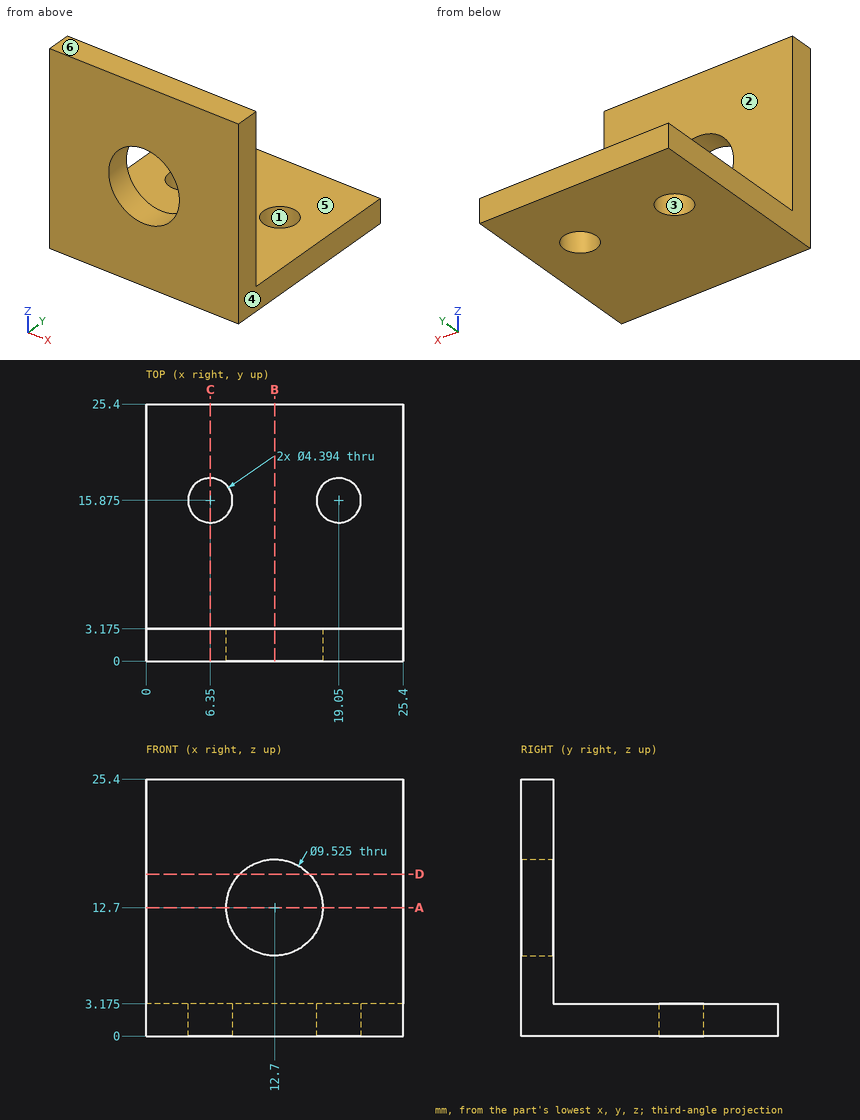
Job drawing, mm, ordinate dimensions from the low corner. One solid piece. A direction names the side the tool comes from. Round coordinates to 2 decimals unless told otherwise and drop trailing zeros. Loops run counter-clockwise (first coordinate to the right, second up) from the corner with the lowest first, then second, coordinate; pieces in that order, holes last.
(1) Two-plate mould, pull along Y, no slides. Class the marked faces 1, 2, 3 and 4: +Y half, -Y half, draft (parallel to the pull), parting line (faces both ways), or undercut.
(2) Cut at C-C (x = 6.35). Give the cut face in (y, z) (1 decimal), plus the area to 3 significant figures.
(3) Drop flat-ended pins along their axis: pin 1 (4 mm diameter, centred on y = 3, z = 6, fed in from -X); pin 2 (3 mm diameter, centred on x = 9.5, z = 11, fed in from +Y) (3 decimals); pin 3 (10 mm diameter, centred on x = 17, y = 16.5, fed in from +Z) (3 decimals). Give the stop position or say it passes through.
(4) Cut at B-B (x = 12.7). Give the cut face in (y, z) (1 decimal), plus the area to 3 significant figures.
(5) Which spindle directions (+Z, -Z, +X, -X, +Y, -Y) get a long thin tool onto all of the face, cutting with end or side? Do the marked faces 5 and 6. Say none if no direction does.
(6) Wall check: line 1 along Y through (x, z) = (6.35, 0.75); line 2 along Z through (x, y) = (12.7, 1.8); line 3 along X through (y, z) = (17.5, 2.25). Give the ranges that are in metal, low to high.
(7) Cut at D-D (z = 16). Give the cut face in (x, y) (1 decimal).
(8) Cut at A-A (z = 12.7). Give the cut face in (x, y) (1 decimal).
Findings below:
1. face 1: undercut
1. face 2: +Y half
1. face 3: undercut
1. face 4: draft
2. outline: (0, 0) - (13.7, 0) - (13.7, 3.2) - (3.2, 3.2) - (3.2, 25.4) - (0, 25.4) - close; (18.1, 0) - (25.4, 0) - (25.4, 3.2) - (18.1, 3.2) - close
2. area: 137 mm2
3. pin 1: stops at x = 0
3. pin 2: stops at y = 3.175
3. pin 3: stops at z = 3.175
4. outline: (0, 0) - (25.4, 0) - (25.4, 3.2) - (3.2, 3.2) - (3.2, 7.9) - (0, 7.9) - close; (0, 17.5) - (3.2, 17.5) - (3.2, 25.4) - (0, 25.4) - close
4. area: 121 mm2
5. face 5: +Z, +X, -X, +Y
5. face 6: +Z, +X, -X, +Y, -Y
6. line 1: y = 0 to 13.68, 18.07 to 25.4
6. line 2: z = 0 to 7.94, 17.46 to 25.4
6. line 3: x = 0 to 4.87, 7.83 to 17.57, 20.53 to 25.4
7. outline: (0, 0) - (9.3, 0) - (9.3, 3.2) - (0, 3.2) - close; (16.1, 0) - (25.4, 0) - (25.4, 3.2) - (16.1, 3.2) - close
8. outline: (0, 0) - (7.9, 0) - (7.9, 3.2) - (0, 3.2) - close; (17.5, 0) - (25.4, 0) - (25.4, 3.2) - (17.5, 3.2) - close
